from build123d import *

# Parameters (mm, degrees)
F0_W     = 609.6
F0_H     = 850.9
F1_DEPTH = 152.4
F2_W     = 609.6
F2_H     = 76.2
F3_DEPTH = 609.6
F4_W     = 76.2
F4_H     = 76.2
F5_DEPTH = 127
F6_R     = 31.75
F7_DEPTH = 137.16
F8_W     = 76.2
F8_H     = 609.6


with BuildPart() as f1:
    # F0 (on Right) → F1 (new body)
    with BuildSketch(Plane.YZ):
        Rectangle(F0_W, F0_H)
    extrude(amount=F1_DEPTH)

    # F2 (on face) → F3 (join)
    with BuildSketch(Plane.YZ.offset(152.4)):
        with Locations((0, -387.35)):
            Rectangle(F2_W, F2_H)
    extrude(amount=F3_DEPTH)

    # F4 (on face) → F5 (join)
    with BuildSketch(Plane.YZ.offset(762)):
        with Locations((0, -387.35)):
            Rectangle(F4_W, F4_H)
    extrude(amount=F5_DEPTH)

    # F6 (on face) → F7 (cut)
    with BuildSketch(Plane.XY.offset(-349.25)):
        with Locations((825.5, 0)):
            Circle(F6_R)
    extrude(amount=-F7_DEPTH, mode=Mode.SUBTRACT)

    # F8 (on face) → F9 (revolve)
    with BuildSketch(Plane.XY.offset(425.45)):
        with Locations((38.1, 0)):
            Rectangle(F8_W, F8_H)
    revolve(axis=Axis((0, 0, 425.45), (0, -1, 0)))


solid = f1.part
Here's how the part is built. I have some questions about the finished solid (model axes, mm). A direction names the side the tool comes from. Coordinates: 2 decimals unless noted, no trailing zeros. Order: outer loops, then holes, each group sorted by start corner. A loop starts at its lowest first (then second) coordinate and runs counter-clockwise, first axis right, second up. Notation, with made-up numbers: M 43,78.5 L 78,78.5 A27 ccw 78,102.5 Z; hole C 43,-33.5 d7. An arc over 180 degrees is marked long. Answer as CSV lines item,"result". Start each with the question number.
1. On a 3-axis mill with a long thin cutter (end or side, diameter ignored), from which of +Z, -Z, +X, -X, +Y, -Y can I reach the whole of each face in a straight line? I mean faces 1 (the flat face through (152.4, -4, 44)), 2 (the flat face through (762, -173, -387)), 3 (the flat face through (825, 38.1, -388)), 4 (the cylindrical face through (-52.075, 4.267, 481.079)). Say none if no direction works.
2. We'd pull the mould along X, two halves only. Please class faces 5 (the flat face through (0, -4, -33)), 6 (the cylindrical face through (855.784, 9.537, -386.817)), 7 (the flat face through (762, 170, -387)): released by +X, released by -X, zero draft, split by the parting line, or undercut.
3. I want a section at C-C, the plane y = 67.5. Write out the boundary of the cut face in (x, z).
4. I need wall thicknesses on line 1 (Y direction, x = 825, z = -385); line 2 (X direction, y = -224, z = 324); line 3 (Z direction, x = 337, y = 118). Which ranges of each line are inside material? Lowest first, please. Write a range as [from, to].
5. I want a section at D-D, the plane z = 268. Write out the boundary of the cut face in (x, y).
6. For pin 1 (23 mm diameter, centred on x = 855, z = -403.5, fed in from +Y); pin 2 (5 mm diameter, centred on x = 220, y = -158, fed in from +Z); pin 3 (23 mm diameter, centred on x = 122, y = -51, fed in from +Z), each with a flat end and sliding along its axis, tell me the tip position at first contact or that it passes through.
7. I want a section at B-B, the plane y = 0. Write out the boundary of the cut face in (x, z).
8. I want a section at A-A, the plane x = 820. Write out the boundary of the cut face in (y, z), and give its area (3 significant figures).
Recorded:
1,face 1,"+Z, +X, +Y, -Y"
1,face 2,"+Z, -Z, +X, -Y"
1,face 3,"+Z, -Z, +X, +Y"
1,face 4,"+Y, -Y"
2,face 5,"released by -X"
2,face 6,"undercut"
2,face 7,"released by +X"
3,outline,"M 0,-425.45 L 762,-425.45 L 762,-349.25 L 152.4,-349.25 L 152.4,425.45 L 76.2,425.45 A76.2 ccw long 0,349.25 Z"
4,line 1,"y = [-38.1, -31.75], [31.75, 38.1]"
4,line 2,"x = [0, 152.4]"
4,line 3,"z = [-425.45, -349.25]"
5,outline,"M 0,-304.8 L 152.4,-304.8 L 152.4,304.8 L 0,304.8 Z"
6,pin 1,"stops at y = 38.1"
6,pin 2,"stops at z = -349.25"
6,pin 3,"stops at z = 425.45"
7,outline,"M 0,-425.45 L 793.75,-425.45 L 793.75,-349.25 L 152.4,-349.25 L 152.4,425.45 L 76.2,425.45 A76.2 ccw long 0,349.25 Z; M 857.25,-425.45 L 889,-425.45 L 889,-349.25 L 857.25,-349.25 Z"
8,outline,"M -38.1,-425.45 L -31.27,-425.45 L -31.27,-349.25 L -38.1,-349.25 Z; M 31.27,-425.45 L 38.1,-425.45 L 38.1,-349.25 L 31.27,-349.25 Z"
8,area,"1,040 mm2"
